from build123d import *

# Parameters (mm, degrees)
BOSS_EXTRUDE1_DEPTH = 200
SHELL1_T            = -17


with BuildPart() as part:
    # Sketch1 → Boss-Extrude1 (new body)
    with BuildSketch(Plane.XY):
        with BuildLine():
            Line((-151.256685576, -7.691916928), (-15.667118089, 27.373929479))
            ThreePointArc((-15.667118089, 27.373929479), (3.41183822, 29.801079282), (22.490794529, 27.373929479))
            Line((22.490794529, 27.373929479), (158.080362016, -7.691916928))
            Line((158.080362016, -7.691916928), (-151.256685576, -7.691916928))
        make_face()
    extrude(amount=BOSS_EXTRUDE1_DEPTH)

    # Shell1
    shell1_openings = [part.faces().sort_by_distance(p)[0] for p in [
        (3.41183822, -7.691916928, 100),
    ]]
    offset(amount=SHELL1_T, openings=shell1_openings, kind=Kind.INTERSECTION)


solid = part.part
Input: part model. Units: mm. Frame: model coordinates. A direction names the side the tool comes from. Round coordinates to 2 decimals unless told otherwise and drop trailing zeros. Order: outer loops, then holes, each group sorted by start corner. A loop starts at its lowest first (then second) coordinate and runs counter-clockwise, first axis right, second up. Notation, with made-up numbers: (85.25, 11) - (102.25, 11) arc R20 cw to (102.25, 19) - close; hole circle Ø4 at (69, -1.5). An arc over 180 degrees is marked (long way). Use a Markdown table: item, result.
1. Mould query, pull axis X, two halves, no side actions, for faces 3 (the face through (6, 7, 0)), 4 (the face through (89.336, 10.086, 98.6)), 5 (the face through (3.2, 12.8, 98.8)). Classes: +X half, -X half, draft (parallel to the pull), parting line (faces both ways), or undercut.
Evaluation:
| item | result |
|---|---|
| face 3 | draft |
| face 4 | +X half |
| face 5 | undercut |
2. Section D-D on x = 109. Return the cut outline in (y, z), then the cut area to 3 significant figures.
Evaluation:
| item | result |
|---|---|
| outline | (-7.69, 0) - (5, 0) - (5, 200) - (-7.69, 200) - close |
| area | 2,540 mm^2 |
3. First-contact query: pin 1 (10 mm diameter, centred on x = 54, z = 72, fed in from +Y); pin 2 (8 mm diameter, centred on x = -60.5, z = 51.5, fed in from -Y); pin 3 (2 mm diameter, centred on x = -8.5, z = 173.5, fed in from +Y). Flat tips, straight axial feed; report the tip coordinate or a pass-through.
Evaluation:
| item | result |
|---|---|
| pin 1 | y = 20.52 |
| pin 2 | y = -2.81 |
| pin 3 | y = 29.02 |
4. Section A-A on y = 6. Return the cut outline in (x, z), then the cut area to 3 significant figures.
Evaluation:
| item | result |
|---|---|
| outline | (-98.31, 0) - (105.14, 0) - (105.14, 200) - (-98.31, 200) - close; hole (-30.42, 17) - (37.24, 17) - (37.24, 183) - (-30.42, 183) - close |
| area | 29,500 mm^2 |
5. Access query for faces 1 (the face through (3.1, 29.8, 98.6)), 2 (the face through (5, 0, 17)). Directions: +Z, -Z, +X, -X, +Y, -Y. A direction counts if a zero-diameter tool reaches every point of the face in a straight line with its end or side. Return the directions, or none.
Evaluation:
| item | result |
|---|---|
| face 1 | +Z, -Z, +Y |
| face 2 | -Y |
6. Material intervals for probe 1 along Z at (x, y) = (-13, 8); probe 2 along Y at (x, z) = (-121, 49); probe 3 along Y at (x, z) = (-46, 12.5), sorted ascending.
Evaluation:
| item | result |
|---|---|
| probe 1 | 0 to 17, 183 to 200 |
| probe 2 | -7.69 to 0.13 |
| probe 3 | -7.69 to 19.53 |
7. Section C-C on z = 87. Return the cut outline in (x, y).
Evaluation:
| item | result |
|---|---|
| outline | (-151.26, -7.69) - (-83.36, -7.69) - (-11.41, 10.92) arc R59.2 cw to (18.23, 10.92) - (90.18, -7.69) - (158.08, -7.69) - (22.49, 27.37) arc R76.2 ccw to (-15.67, 27.37) - close |
8. Section B-B on x = 59. Return the cut outline in (y, z).
Evaluation:
| item | result |
|---|---|
| outline | (-7.69, 0) - (17.93, 0) - (17.93, 200) - (-7.69, 200) - (-7.69, 183) - (0.37, 183) - (0.37, 17) - (-7.69, 17) - close |
